Can you work these out from the model? Positions are in its coordinate system, mm. Face numbers are marked on the shaded views. A direction names the side the tool comes from. Round coordinates to 2 decimals unless told otherwise and drop trailing zeros. One line per item, written item: value.
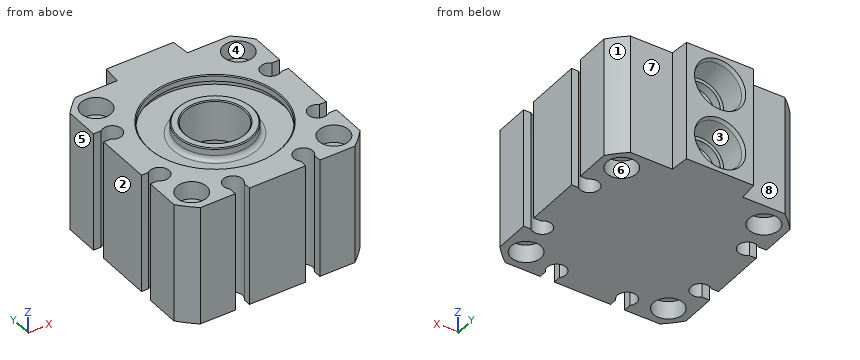
```python
from build123d import *

# Parameters (mm, degrees)
EXTRUDE1_DEPTH                               = 12.7635
EXTRUDE1_DEPTH_BACK                          = 12.7635
SKETCH1_W                                    = 39.69
SKETCH1_H                                    = 39.69
F_056_250_NOSE_CHAMFER_R                     = 1
SKETCH13_R                                   = 28.065068145
SKETCH13_R_2                                 = 25.795
F_075_250_TUBE_EDGE_ROUNDOVER_DEPTH          = 38.937788272
F_075_250_PORT_BOSS_DEPTH                    = 25.527
F_106_200_PORT_1_8_NPT_AT_2_COUNT            = 2
F_106_200_PORT_1_8_NPT_AT_2_PITCH            = 12.827
F_075_250_SWITCH_GROOVE_DEPTH                = 41.157265582
F_075_106_SWITCH_GROOVE_CIRC_PATTERN_COUNT   = 3
F_075_106_SWITCH_GROOVE_CIRC_PATTERN_ANGLE   = 180
SKETCH19_W                                   = 0.15
SKETCH19_H                                   = 12
F_075_250_THIN_SIDE_CUTS_DEPTH               = 41.157265582
SKETCH20_R                                   = 1.95
F_075_250_MOUNT_THRU_HOLE_DEPTH              = 41.157265582
F_075_250_MOUNT_THRU_HOLE_CIRC_PATTERN_COUNT = 4
SKETCH21_R                                   = 3.175
F_075_250_B_MOUNT_CBORE_ROD_END_DEPTH        = 3.81
F_056_250_START                              = -4.0875
SKETCH22_R                                   = 13.462
F_056_250_STROKE_CHAMBER_DEPTH               = 8.175
SKETCH23_R                                   = 6.35
F_056_250_ROD_THRU_BORE_DEPTH                = 34.524396822
F_056_250_COLLAR_CHAMFER_SIZE                = 0.2


with BuildPart() as part:
    # Sketch1 → Extrude1 (new, two sides: drawn at the far end of the back side and taken through both)
    with BuildSketch(Plane.XY.offset(-EXTRUDE1_DEPTH_BACK)):
        Rectangle(SKETCH1_W, SKETCH1_H)
    extrude(amount=EXTRUDE1_DEPTH + EXTRUDE1_DEPTH_BACK)

    # Sketch33 → 056-250 Front Recess (revolve, cut)
    with BuildSketch(Plane(origin=(0, 0, 0), x_dir=(0, 0, -1), z_dir=(1, 0, 0)), mode=Mode.PRIVATE) as f_056_250_front_recess_sk:
        Polygon((-12.7635, 14), (-11.4135, 14), (-11.4135, 14.7), (-10.2385, 14.7), (-10.2385, 8), (-12.7635, 8), align=None)
    revolve(f_056_250_front_recess_sk.sketch.rotate(Axis((0, 0, 61.220394237), (0, 0, -1)), 90), axis=Axis((0, 0, 61.220394237), (0, 0, -1)), mode=Mode.SUBTRACT)

    # 056-250 Nose Chamfer
    f_056_250_nose_chamfer_edges = [part.edges().sort_by_distance(p)[0] for p in [
        (-8, 0, 10.2385),
    ]]
    fillet(f_056_250_nose_chamfer_edges, radius=F_056_250_NOSE_CHAMFER_R)

    # Sketch13 → 075-250 Tube Edge Roundover (cut, through all)
    with BuildSketch(Plane.XY.offset(12.7635)):
        Circle(SKETCH13_R)
        Circle(SKETCH13_R_2, mode=Mode.SUBTRACT)
    extrude(amount=-F_075_250_TUBE_EDGE_ROUNDOVER_DEPTH, mode=Mode.SUBTRACT)

    # Sketch14 → 075-250 Port Boss (add)
    with BuildSketch(Plane.XY.offset(12.7635)):
        Polygon((-7.15, 23.815), (7.15, 23.815), (7.497329994, 19.845), (-7.497329994, 19.845), align=None)
    extrude(amount=-F_075_250_PORT_BOSS_DEPTH)

    # Sketch36 → 106-200 Port 1/8 NPT (revolve, cut)
    with BuildSketch(Plane(origin=(0, 23.815, 6.4135), x_dir=(0, 0, 1), z_dir=(1, 0, 0))):
        Polygon((0, 0), (0, 10.533468714), (4.2164, 8), (4.2164, 6.2), (4.959907269, 6.2), (5.1218211, 0.792298297), (5.4500018, 0), align=None)
    f_106_200_port_1_8_npt = revolve(axis=Axis((0, 30.165, 6.4135), (0, -1, 0)), mode=Mode.SUBTRACT)

    # 106-200 Port 1/8 NPT at 2: 106-200 Port 1/8 NPT ×2
    with Locations(*[(0, 0, -i * F_106_200_PORT_1_8_NPT_AT_2_PITCH) for i in range(1, F_106_200_PORT_1_8_NPT_AT_2_COUNT)]):
        add(f_106_200_port_1_8_npt, mode=Mode.SUBTRACT)

    # Sketch15 → 075-250 Switch Groove (cut, through all)
    with BuildSketch(Plane.XY.offset(12.7635)):
        with BuildLine():
            Line((-19.845, 9), (-18.205376786, 9))
            ThreePointArc((-18.205376786, 9), (-14.82, 7.5), (-18.205376786, 6))
            Line((-18.205376786, 6), (-19.845, 6))
            Line((-19.845, 6), (-19.845, 9))
        make_face()
        with BuildLine():
            Line((-19.845, -9), (-19.845, -6))
            Line((-19.845, -6), (-18.205376786, -6))
            ThreePointArc((-18.205376786, -6), (-14.82, -7.5), (-18.205376786, -9))
            Line((-18.205376786, -9), (-19.845, -9))
        make_face()
    f_075_250_switch_groove = extrude(amount=-F_075_250_SWITCH_GROOVE_DEPTH, mode=Mode.SUBTRACT)

    # 075-106 Switch Groove Circ Pattern: 075-250 Switch Groove ×3 about axis
    f_075_106_switch_groove_circ_pattern_axis = Axis((0, 0, 0), (0, 0, 1))
    for i in range(1, F_075_106_SWITCH_GROOVE_CIRC_PATTERN_COUNT):
        add(f_075_250_switch_groove.rotate(f_075_106_switch_groove_circ_pattern_axis, i * F_075_106_SWITCH_GROOVE_CIRC_PATTERN_ANGLE / (F_075_106_SWITCH_GROOVE_CIRC_PATTERN_COUNT - 1)), mode=Mode.SUBTRACT)

    # Sketch19 → 075-250 Thin Side Cuts (cut, through all)
    with BuildSketch(Plane.XY.offset(12.7635)):
        with Locations((19.77, 0)):
            Rectangle(SKETCH19_W, SKETCH19_H)
        with Locations((-19.77, 0)):
            Rectangle(SKETCH19_W, SKETCH19_H)
    extrude(amount=-F_075_250_THIN_SIDE_CUTS_DEPTH, mode=Mode.SUBTRACT)

    # Sketch20 → 075-250 Mount Thru Hole (cut, through all)
    with BuildSketch(Plane.XY.offset(12.7635)):
        with Locations((15.155, 15.155)):
            Circle(SKETCH20_R)
    f_075_250_mount_thru_hole = extrude(amount=-F_075_250_MOUNT_THRU_HOLE_DEPTH, mode=Mode.SUBTRACT)

    # 075-250 Mount Thru Hole Circ Pattern: 075-250 Mount Thru Hole ×4 about axis
    f_075_250_mount_thru_hole_circ_pattern_axis = Axis((0, 0, 0), (0, 0, 1))
    for i in range(1, F_075_250_MOUNT_THRU_HOLE_CIRC_PATTERN_COUNT):
        add(f_075_250_mount_thru_hole.rotate(f_075_250_mount_thru_hole_circ_pattern_axis, i * 360 / F_075_250_MOUNT_THRU_HOLE_CIRC_PATTERN_COUNT), mode=Mode.SUBTRACT)

    # Sketch21 → 075-250 B Mount CBore Rod End (cut)
    with BuildSketch(Plane.XY.offset(12.7635)):
        with Locations((-15.155, 15.155)):
            Circle(SKETCH21_R)
        with Locations((-15.155, -15.155)):
            Circle(SKETCH21_R)
        with Locations((15.155, 15.155)):
            Circle(SKETCH21_R)
        with Locations((15.155, -15.155)):
            Circle(SKETCH21_R)
    f_075_250_b_mount_cbore_rod_end = extrude(amount=-F_075_250_B_MOUNT_CBORE_ROD_END_DEPTH, mode=Mode.SUBTRACT)

    # 075-250 B Mount CBore Non-Rod End: 075-250 B Mount CBore Rod End across plane
    add(f_075_250_b_mount_cbore_rod_end.mirror(Plane.XY), mode=Mode.SUBTRACT)

    # Sketch22 → 056-250 Stroke Chamber (cut)
    with BuildSketch(Plane.XY.offset(F_056_250_START)):
        Circle(SKETCH22_R)
    extrude(amount=F_056_250_STROKE_CHAMBER_DEPTH, mode=Mode.SUBTRACT)

    # Sketch23 → 056-250 Rod Thru Bore (cut, through all)
    with BuildSketch(Plane.XY):
        Circle(SKETCH23_R)
    extrude(amount=F_056_250_ROD_THRU_BORE_DEPTH, mode=Mode.SUBTRACT)

    # 056-250 Collar Chamfer
    f_056_250_collar_chamfer_edges = [part.edges().sort_by_distance(p)[0] for p in [
        (-14, 0, 12.7635),
        (-8, 0, 12.7635),
        (-6.35, 0, 12.7635),
    ]]
    chamfer(f_056_250_collar_chamfer_edges, length=F_056_250_COLLAR_CHAMFER_SIZE)


solid = part.part
```
Q1. Please list where these lines run through material, in increasing order: line 1 along Z through (x, y) = (0, 16.7); line 2 along X through (y, z) = (16, -5.75) (3 decimals); line 3 along Y through (x, z) = (16, 0) (3 decimals).
Answers below:
line 1: -12.76 to -10.63, -2.2 to 2.2, 10.63 to 12.76
line 2: -19.845 to -16.912, -13.398 to -4.164, 4.164 to 13.398, 16.912 to 19.845
line 3: -19.845 to -16.912, -13.398 to -9.34, -5.66 to 5.66, 9.34 to 13.398, 16.912 to 19.845
Q2. Will these pins go through, and if not, where does the flat tip stop? pin 1 Ø7 at (x, y) = (-15.5, 15.5) entering from -Z; pin 2 Ø1 at (x, y) = (-6, 12) entering from +Z; pin 3 Ø4 at (x, z) = (2.5, 6.5) entering from +Y (3 decimals); pin 4 Ø5 at (x, z) = (11.5, -9) entering from +Y (3 decimals).
Answers below:
pin 1: z = -12.76
pin 2: z = 10.24
pin 3: y = 17.615
pin 4: y = 19.845
Q3. On a 3-axis mill with a long thin cutter (end or side, diameter ignored), from which of +Z, -Z, +X, -X, +Y, -Y can I reach the whole of each face in a straight line? I mean the marked faces 4, 5, 6, 7 and 8. Say none if no direction works.
Answers below:
face 4: +Z
face 5: +Z, -Z, -X, +Y, -Y
face 6: -Z
face 7: +Z, -Z, +X, +Y
face 8: +Z, -Z, -X, +Y
Q4. We'd pull the mould along X, two halves only. Please class the marked faces 1, 2 and 3: released by +X, released by -X, zero draft, split by the parting line, or undercut.
Answers below:
face 1: released by +X
face 2: released by -X
face 3: undercut
Q5. I want a section at B-B on z = -8. Give the number of separate pieces and of enclosed holes in the cut face, plus the area to 3 significant figures.
Answers below:
separate pieces: 1
enclosed holes: 4
area: 1,380 mm^2
